Read the model definition and answer for the solid it produces. Units are mm, in the model's axes. Coordinates: 2 decimals unless noted, no trailing zeros. Write each loop counter-clockwise with the first axis right and the second up, starting at its lowest first coordinate (ties: lowest second). Pieces come first, ordered by that corner, then holes. Notation, with made-up numbers: (37, -24) -> (82, -24) arc R32 ccw to (82, 8) -> close; hole circle Ø5 at (-22.5, 1). An arc over 180 degrees is marked (long way). Return JSON: item names as keys, results as strings.
from build123d import *

# Parameters (mm, degrees)
SKETCH_W       = 190
SKETCH_H       = 82
SKETCH_R       = 1.65
PAD_DEPTH      = 0.75
PAD_DEPTH_BACK = 0.75
SKETCH001_R    = 15
POCKET_DEPTH   = 1.501


with BuildPart() as part:
    # Sketch → Pad (new body, two sides)
    with BuildSketch(Plane.XZ) as pad_sk:
        Rectangle(SKETCH_W, SKETCH_H)
        with Locations((90, 30)):
            Circle(SKETCH_R, mode=Mode.SUBTRACT)
        with Locations((90, 10)):
            Circle(SKETCH_R, mode=Mode.SUBTRACT)
        with Locations((90, -30)):
            Circle(SKETCH_R, mode=Mode.SUBTRACT)
        with Locations((90, -10)):
            Circle(SKETCH_R, mode=Mode.SUBTRACT)
        with Locations((-90, 30)):
            Circle(SKETCH_R, mode=Mode.SUBTRACT)
        with Locations((-90, 10)):
            Circle(SKETCH_R, mode=Mode.SUBTRACT)
        with Locations((-90, -30)):
            Circle(SKETCH_R, mode=Mode.SUBTRACT)
        with Locations((-90, -10)):
            Circle(SKETCH_R, mode=Mode.SUBTRACT)
    extrude(amount=PAD_DEPTH)
    extrude(pad_sk.sketch, amount=-PAD_DEPTH_BACK)

    # Sketch001 (on Face14 of Pad) → Pocket (cut, through all)
    with BuildSketch(Plane.XZ.offset(0.75)):
        with Locations((-17.2, -17.5)):
            Circle(SKETCH001_R)
        with Locations((17.2, -17.5)):
            Circle(SKETCH001_R)
    extrude(amount=-POCKET_DEPTH, mode=Mode.SUBTRACT)


solid = part.part
1. For a pull along X with two mould halves and no side action, classify faces 1 (the face through (-28.256, -0.01, -7.362)), 2 (the face through (-1, 0.75, 1)) as +X half, -X half, draft (parallel to the pull), parting line (faces both ways), or undercut.
Taken from the geometry:
{"face 1": "undercut", "face 2": "draft"}
2. The part is cut by section B-B (z = -17.5). Determine the outline of the cut face in (x, y).
Taken from the geometry:
{"outline": "(-95, -0.75) -> (-32.2, -0.75) -> (-32.2, 0.75) -> (-95, 0.75) -> close; (-2.2, -0.75) -> (2.2, -0.75) -> (2.2, 0.75) -> (-2.2, 0.75) -> close; (32.2, -0.75) -> (95, -0.75) -> (95, 0.75) -> (32.2, 0.75) -> close"}
3. The part is cut by section C-C (x = 13.5). Determine the outline of the cut face in (y, z).
Taken from the geometry:
{"outline": "(-0.75, -41) -> (0.75, -41) -> (0.75, -32.04) -> (-0.75, -32.04) -> close; (-0.75, -2.96) -> (0.75, -2.96) -> (0.75, 41) -> (-0.75, 41) -> close"}
4. Flat-ended cylindrical pins translate along their axes: pin 1 Ø3 at (x, z) = (-90, -10) entering from -Y; pin 2 Ø4 at (x, z) = (90, 30) entering from -Y. Find the tip coordinate at first contact, or state that the pin passes through.
Taken from the geometry:
{"pin 1": "passes through", "pin 2": "stops at y = -0.75"}
5. The part is cut by section D-D (x = -19). Determine the outline of the cut face in (y, z).
Taken from the geometry:
{"outline": "(-0.75, -41) -> (0.75, -41) -> (0.75, -32.39) -> (-0.75, -32.39) -> close; (-0.75, -2.61) -> (0.75, -2.61) -> (0.75, 41) -> (-0.75, 41) -> close"}
6. Consider L1, parallel to Z at x = -90, y = 0.4; L2, parallel to Z at x = -17.2, y = -0.35; L3, parallel to Z at x = 21, y = -0.6. Determine where each line is inside the solid, lowest interval first.
Taken from the geometry:
{"L1": "z = -41 to -31.65, -28.35 to -11.65, -8.35 to 8.35, 11.65 to 28.35, 31.65 to 41", "L2": "z = -41 to -32.5, -2.5 to 41", "L3": "z = -41 to -32.01, -2.99 to 41"}
7. The part is cut by section A-A (y = 0.3). Count the separate pieces of the cut face and the enclosed holes in it, then the cut area to 3 significant figures.
Taken from the geometry:
{"separate pieces": "1", "enclosed holes": "10", "area": "14,100 mm2"}
